from build123d import *

# Parameters (mm, degrees)
SKETCH4_R            = 55.88
BOSS_EXTRUDE2_DEPTH  = 10.16
BOSS_EXTRUDE4_DEPTH  = 101.6
BOSS_EXTRUDE5_DEPTH  = 9.525
BOSS_EXTRUDE6_START  = -9.525
BOSS_EXTRUDE6_DEPTH  = 9.525
CUT_EXTRUDE4_REACH   = 223.16
SKETCH12_R           = 21.5
SKETCH13_W           = 38.1
SKETCH13_H           = 69.85
CUT_EXTRUDE5_DEPTH   = 76.2
BOSS_EXTRUDE10_DEPTH = 19.05
SKETCH28_R           = 11.2395
CUT_EXTRUDE9_DEPTH   = 38.1
CUT_EXTRUDE10_DEPTH  = 7.366
CHAMFER1_SIZE        = 6.35
SKETCH30_R           = 2.1
CUT_EXTRUDE11_DEPTH  = 7.366
SKETCH31_R           = 3.175
CUT_EXTRUDE12_DEPTH  = 223.900333216
BOSS_EXTRUDE11_DEPTH = 38.1
CHAMFER2_SIZE        = 25.4
CUT_EXTRUDE13_REACH  = 233.204
SKETCH34_R           = 3.175
SKETCH35_R           = 3.175
CUT_EXTRUDE14_DEPTH  = 246.746626534
SKETCH36_W           = 63.5
SKETCH36_H           = 36.709955102
CUT_EXTRUDE15_DEPTH  = 63.5
FILLET1_R            = 6.35
SKETCH37_W           = 210.742334846
SKETCH37_H           = 201.224939079
CUT_EXTRUDE16_DEPTH  = 232.093968202


with BuildPart() as part:
    # Sketch4 → Boss-Extrude2 (new body)
    with BuildSketch(Plane(origin=(0, 0, 0), x_dir=(1, 0, 0), z_dir=(0, 1, 0))):
        with Locations(Location((0, 0, 0), (0, 0, 270))):
            Circle(SKETCH4_R)
    extrude(amount=BOSS_EXTRUDE2_DEPTH)

    # Sketch8 → Boss-Extrude4 (add)
    with BuildSketch(Plane(origin=(0, 10.16, 0), x_dir=(1, 0, 0), z_dir=(0, 1, 0))):
        Polygon((0, 43.994090512), (-38.1, 21.997045256), (-38.1, -21.997045256), (0, -43.994090512), (38.1, -21.997045256), (38.1, 21.997045256), align=None)
    extrude(amount=BOSS_EXTRUDE4_DEPTH)

    # Sketch9 → Boss-Extrude5 (add)
    with BuildSketch(Plane(origin=(-19.05, 0, -32.995567884), x_dir=(-0.8660254037844386, 0, 0.5000000000000003), z_dir=(-0.5000000000000002, 0, -0.8660254037844385))):
        with BuildLine():
            Line((21.997045256, 111.76), (-21.997045256, 111.76))
            Line((-21.997045256, 111.76), (-21.997045256, 124.225996336))
            ThreePointArc((-21.997045256, 124.225996336), (0, 188.144153123), (21.997045256, 124.225996336))
            Line((21.997045256, 124.225996336), (21.997045256, 111.76))
        make_face()
    extrude(amount=-BOSS_EXTRUDE5_DEPTH)

    # Sketch10 → Boss-Extrude6 (add)
    with BuildSketch(Plane(origin=(19.05, 0, 32.995567884), x_dir=(0.8660254037844386, 0, -0.5000000000000001), z_dir=(0.5000000000000001, 0, 0.8660254037844386)).offset(BOSS_EXTRUDE6_START)):
        with BuildLine():
            Line((-21.997045256, 111.76), (21.997045256, 111.76))
            Line((21.997045256, 111.76), (21.997045256, 124.225996336))
            ThreePointArc((21.997045256, 124.225996336), (0, 188.144153123), (-21.997045256, 124.225996336))
            Line((-21.997045256, 124.225996336), (-21.997045256, 111.76))
        make_face()
    extrude(amount=BOSS_EXTRUDE6_DEPTH)

    # Cut-Extrude4: up to this face of the body (flat: up to its plane)
    cut_extrude4_end = Plane(part.part.faces().sort_by_distance((19.05, 104.643172711, 32.995567884))[0])
    # Sketch12 → Cut-Extrude4 (cut, up to the picked face)
    with BuildSketch(Plane(origin=(-19.05, 0, -32.995567884), x_dir=(-0.8660254037844386, 0, 0.5000000000000003), z_dir=(-0.5000000000000002, 0, -0.8660254037844385)), mode=Mode.PRIVATE) as cut_extrude4_sk1:
        with Locations((0, 152.4)):
            Circle(SKETCH12_R)
    cut_extrude4_tool1 = split(extrude(cut_extrude4_sk1.sketch, amount=-CUT_EXTRUDE4_REACH, mode=Mode.PRIVATE), bisect_by=cut_extrude4_end, keep=Keep.BOTH, mode=Mode.PRIVATE)
    add(cut_extrude4_tool1.solids().sort_by(Axis((-19.05, 152.4, -32.995568), (0.5000000000000002, 0, 0.8660254037844385)))[0], mode=Mode.SUBTRACT)

    # Sketch13 → Cut-Extrude5 (cut, symmetric)
    with BuildSketch(Plane(origin=(-19.05, 0, 10.998522628), x_dir=(0.5000000000000002, 0, 0.8660254037844386), z_dir=(-0.8660254037844385, 0, 0.5000000000000001))):
        with Locations((0, 76.835)):
            Rectangle(SKETCH13_W, SKETCH13_H)
    extrude(amount=CUT_EXTRUDE5_DEPTH, both=True, mode=Mode.SUBTRACT)

    # Sketch22 → Boss-Extrude10 (add, symmetric)
    with BuildSketch(Plane(origin=(0, 0, 0), x_dir=(-0.8660254037844386, 0, 0.5000000000000001), z_dir=(-0.5000000000000001, 0, -0.8660254037844386))):
        with BuildLine():
            Line((43.994090512, 41.91), (102.10102108, 41.91))
            ThreePointArc((102.10102108, 41.91), (117.97602108, 26.035), (102.10102108, 10.16))
            Line((102.10102108, 10.16), (43.994090512, 10.16))
            Line((43.994090512, 10.16), (21.997045256, 10.16))
            Line((21.997045256, 10.16), (21.997045256, 41.91))
            Line((21.997045256, 41.91), (43.994090512, 41.91))
        make_face()
    extrude(amount=BOSS_EXTRUDE10_DEPTH, both=True)

    # Sketch28 → Cut-Extrude9 (cut)
    with BuildSketch(Plane(origin=(9.525, 0, 16.497783942), x_dir=(0.8660254037844386, 0, -0.5000000000000001), z_dir=(0.5000000000000001, 0, 0.8660254037844386))):
        with Locations((-102.10102108, 26.035)):
            Circle(SKETCH28_R)
    extrude(amount=-CUT_EXTRUDE9_DEPTH, mode=Mode.SUBTRACT)

    # Sketch29 → Cut-Extrude10 (cut)
    with BuildSketch(Plane(origin=(9.525, 0, 16.497783942), x_dir=(0.8660254037844386, 0, -0.5000000000000001), z_dir=(0.5000000000000001, 0, 0.8660254037844386))):
        with BuildLine():
            Line((-115.737415068, 17.907), (-109.863879848, 17.907))
            ThreePointArc((-109.863879848, 17.907), (-113.34052108, 26.035), (-109.863879848, 34.163))
            Line((-109.863879848, 34.163), (-115.737415068, 34.163))
            ThreePointArc((-115.737415068, 34.163), (-117.97602108, 26.035), (-115.737415068, 17.907))
        make_face()
    extrude(amount=-CUT_EXTRUDE10_DEPTH, mode=Mode.SUBTRACT)

    # Chamfer1
    chamfer1_edges = [part.edges().sort_by_distance(p)[0] for p in [
        (38.1, 41.91, -10.998522628),
        (28.575, 41.91, -27.49630657),
    ]]
    chamfer(chamfer1_edges, length=CHAMFER1_SIZE)

    # Sketch30 → Cut-Extrude11 (cut)
    with BuildSketch(Plane(origin=(0, 41.91, 0), x_dir=(1, 0, 0), z_dir=(0, 1, 0))):
        with Locations(Location((-88.422078008, -51.05051054, 0), (0, 0, 270))):
            Circle(SKETCH30_R)
    extrude(amount=-CUT_EXTRUDE11_DEPTH, mode=Mode.SUBTRACT)

    # Sketch31 → Cut-Extrude12 (cut, through all)
    with BuildSketch(Plane(origin=(0, 10.16, 0), x_dir=(1, 0, 0), z_dir=(0, 1, 0))):
        with Locations(Location((-49.089000823, 6.594762938, 0), (0, 0, 270))):
            Circle(SKETCH31_R)
        with Locations(Location((26.925278647, 41.57222955, 0), (0, 0, 270))):
            Circle(SKETCH31_R)
    cut_extrude12 = extrude(amount=-CUT_EXTRUDE12_DEPTH, mode=Mode.SUBTRACT)

    # Mirror1: Cut-Extrude12 across plane
    add(cut_extrude12.mirror(Plane(origin=(0, 0, 0), x_dir=(-0.8660254037844386, 0, 0.5000000000000001), z_dir=(-0.5000000000000001, 0, -0.8660254037844386))), mode=Mode.SUBTRACT)

    # Sketch33 → Boss-Extrude11 (add)
    with BuildSketch(Plane(origin=(0, 41.91, 0), x_dir=(1, 0, 0), z_dir=(0, 1, 0))):
        with BuildLine():
            Line((-43.411916389, -22.079834386), (-63.092428819, -33.442383535))
            Line((-63.092428819, -33.442383535), (-61.800298466, -35.680418955))
            Line((-61.800298466, -35.680418955), (-60.542722832, -37.858603849))
            Line((-60.542722832, -37.858603849), (-40.91541904, -26.504074545))
            ThreePointArc((-40.91541904, -26.504074545), (-33.742060338, -19.539834386), (-43.411916389, -22.079834386))
        make_face()
    extrude(amount=BOSS_EXTRUDE11_DEPTH)

    # Chamfer2
    chamfer2_edges = [part.edges().sort_by_distance(p)[0] for p in [
        (-61.817575825, 80.01, 35.650493692),
    ]]
    chamfer(chamfer2_edges, length=CHAMFER2_SIZE)

    # Cut-Extrude13: up to this plane
    cut_extrude13_end = Plane(origin=(-60.542722832, 80.01, 37.858603849), z_dir=(-0.500750644235671, 0, -0.8655915851587056))
    # Sketch34 → Cut-Extrude13 (cut, up to the surface)
    with BuildSketch(Plane(origin=(-1.292130352, 0, -2.23803542), x_dir=(-0.8660254037844386, 0, 0.5000000000000003), z_dir=(-0.5000000000000002, 0, -0.8660254037844385)), mode=Mode.PRIVATE) as cut_extrude13_sk1:
        with Locations((55.184849848, 61.159110234)):
            Circle(SKETCH34_R)
    cut_extrude13_tool1 = split(extrude(cut_extrude13_sk1.sketch, amount=-CUT_EXTRUDE13_REACH, mode=Mode.PRIVATE), bisect_by=cut_extrude13_end, keep=Keep.BOTH, mode=Mode.PRIVATE)
    add(cut_extrude13_tool1.solids().sort_by_distance((-49.083612, 61.15911, 25.35439))[0], mode=Mode.SUBTRACT)

    # Sketch35 → Cut-Extrude14 (cut, through all)
    with BuildSketch(Plane(origin=(19.05, 0, 32.995567884), x_dir=(0.8660254037844386, 0, -0.5000000000000001), z_dir=(0.5000000000000001, 0, 0.8660254037844386))):
        with Locations((0, 23.280078313)):
            Circle(SKETCH35_R)
    extrude(amount=-CUT_EXTRUDE14_DEPTH, mode=Mode.SUBTRACT)

    # Sketch36 → Cut-Extrude15 (cut, symmetric)
    with BuildSketch(Plane(origin=(-19.05, 0, 10.998522628), x_dir=(0.5000000000000004, 0, 0.8660254037844384), z_dir=(-0.8660254037844384, 0, 0.5000000000000004))):
        with Locations((0, 174.660846527)):
            Rectangle(SKETCH36_W, SKETCH36_H)
    extrude(amount=CUT_EXTRUDE15_DEPTH, both=True, mode=Mode.SUBTRACT)

    # Fillet1
    # the kernel refuses this fillet: 6.35 mm, written as the material it takes off along each edge
    with BuildSketch(Plane(origin=(12.272597523, 156.305868976, -21.027711652), x_dir=(0.04103819462533737, -0.9988766133891899, -0.023693412713994805), z_dir=(-0.5000000000000003, 0, -0.8660254037844386))) as fillet1_piece_1:
        with BuildLine():
            CenterArc((6.655634068, -6.291985478), FILLET1_R, 97.750867839, 84.965214409)
            Line((0.312767573, -6.592891819), (0, 0))
            ThreePointArc((0, 0), (2.899617679, -0.196427123), (5.799235358, 0))
        make_face()
    extrude(amount=19.675766287, mode=Mode.SUBTRACT)
    with BuildSketch(Plane(origin=(-24.346831236, 156.305868976, 0.114525399), x_dir=(-0.04103819462533767, -0.9988766133891899, 0.023693412713994975), z_dir=(-0.5000000000000003, 0, -0.8660254037844386))) as fillet1_piece_2:
        with BuildLine():
            CenterArc((6.655634068, 6.291985478), FILLET1_R, 177.283917752, 84.965214409)
            Line((0.312767573, 6.592891819), (0, 0))
            ThreePointArc((0, 0), (2.899617679, 0.196427123), (5.799235358, 0))
        make_face()
    extrude(amount=19.675766287, mode=Mode.SUBTRACT)
    with BuildSketch(Plane(origin=(-14.894977291, 156.305868976, 45.261361242), x_dir=(-0.011364190914464473, -0.999913899736612, 0.0065611186835884), z_dir=(-0.5000000000000002, 0, -0.8660254037844386)), Plane(origin=(-36.459231913, 156.305868976, 7.91097661), x_dir=(-0.011364190914463116, -0.999913899736612, 0.0065611186835876165), z_dir=(-0.5000000000000002, 0, -0.8660254037844386))) as fillet1_piece_3:
        with BuildLine():
            CenterArc((6.26760006, -6.320536654), FILLET1_R, 84.478464497, 94.769665105)
            Line((-0.081853204, -6.237210446), (0, 0))
            ThreePointArc((0, 0), (3.439298151, 0.165849191), (6.878596303, 0))
        make_face()
    extrude(amount=20.371490756, mode=Mode.SUBTRACT)
    with BuildSketch(Plane(origin=(25.080722669, 156.305868976, -27.619132734), x_dir=(0.011364190914465366, -0.999913899736612, -0.00656111868358885), z_dir=(-0.5000000000000002, 0, -0.8660254037844386)), Plane(origin=(46.644977291, 156.305868976, 9.731251898), x_dir=(0.011364190914466365, -0.999913899736612, -0.006561118683589426), z_dir=(-0.5000000000000002, 0, -0.8660254037844386))) as fillet1_piece_4:
        with BuildLine():
            CenterArc((6.26760006, 6.320536654), FILLET1_R, 180.751870398, 94.769665105)
            Line((-0.081853204, 6.237210446), (0, 0))
            ThreePointArc((0, 0), (3.439298151, -0.165849191), (6.878596303, 0))
        make_face()
    extrude(amount=20.371490756, mode=Mode.SUBTRACT)

    # Sketch37 → Cut-Extrude16 (cut, through all)
    with BuildSketch(Plane(origin=(0, 0, 0), x_dir=(-0.8660254037844386, 0, 0.5000000000000001), z_dir=(-0.5000000000000001, 0, -0.8660254037844386))):
        with Locations((30.487295463, 97.29801522)):
            Rectangle(SKETCH37_W, SKETCH37_H)
    extrude(amount=-CUT_EXTRUDE16_DEPTH, mode=Mode.SUBTRACT)


solid = part.part
Work out the finished part from the listing and answer in its coordinate system (mm). A direction names the side the tool comes from. Give positions to 0.01 mm unless a question says otherwise; leave off trailing zeros. Order: outer loops, then holes, each group sorted by start corner. A loop starts at its lowest first (then second) coordinate and runs counter-clockwise, first axis right, second up. Notation, with made-up numbers: (85.5, 44.25) - (138.5, 44.25) arc R20 cw to (138.5, 71.25) - close; hole circle Ø4 at (31, -36). An arc over 180 degrees is marked (long way). Answer as CSV lines item,"result". Start each with the question number.
Q1. For faces 1 (the face through (-14.72, 129.395, -24.497)), 2 (the face through (-38, 80.01, 19)), 3 (the face through (-50.93, 55.44, 26.42)), 4 (the face through (-39.489, 60.693, 17.064)), determine the directions among +Z, -Z, +X, -X, +Y, -Y from which every point of the face is accessible in a straight line to the end or side of a thin tool.
Q2. The part is cut by section C-C (x = 34). Write down the section's boundary in (y, z).
Q3. The part is cut by section B-B (y = 115.5). Write down the section's boundary in (x, z).
Q4. The mould has two halves that part along X. Classify faces 5 (the face through (-26.869, 5.009, -48.996)), 6 (the face through (-106.996, 26.384, 50.622)), 7 (the face through (-45.94, 5.15, -7.01)): +X half, -X half, draft (parallel to the pull), parting line (faces both ways), or undercut.
Q5. The part is cut by section D-D (y = 167). Write down the section's boundary in (x, z).
Q6. Find the intervals of material crossed by L1, parallel to Y at x = -42.5, z = -16.5; L2, parallel to Y at x = -54, z = -9.5; L3, parallel to Y at x = -14.5, z = -9.5, in increasing order. Write a range as [from, to].
Q7. Given pin 1 Ø2.5 at (x, z) = (-40, -11.5) entering from +Y; pin 2 Ø3 at (y, z) = (46, 22) entering from -X; pin 3 Ø5 at (y, z) = (32.5, 42) entering from -X, each flat-ended and moving along its own axis, determine where each tip first touches the part or whether it passes through.
Q8. The part is cut by section A-A (y = 73). Write down the section's boundary in (x, z).
Check result:
1,face 1,"+Z, +X, +Y"
1,face 2,"+Z, +X, -X, +Y"
1,face 3,"-Z, -X, +Y"
1,face 4,"+Y"
2,outline,"(0, -44.35) - (10.16, -44.35) - (10.16, -24.36) - (35.56, -24.36) - (39.66, -19.63) - (0, -19.63) - close"
3,outline,"(-38.1, -22) - (0, -43.99) - (4.76, -35.75) - (-33.34, -13.75) - close"
4,face 5,"parting line"
4,face 6,"-X half"
4,face 7,"undercut"
5,outline,"(-47.31, -16.68) - (-32.72, -25.1) - (-29.54, -19.61) - (-44.13, -11.18) - close; (-5.38, -40.89) - (9.21, -49.31) - (12.38, -43.81) - (-2.21, -35.39) - close"
6,L1,"y = [0, 10.16], [130.9, 173.9]"
6,L2,"y = [0, 10.16]"
6,L3,"y = [0, 41.91]"
7,pin 1,"stops at y = 156.31"
7,pin 2,"stops at x = -45.87"
7,pin 3,"stops at x = -111.26"
8,outline,"(-47.17, 24.25) - (-43.41, 22.08) arc R5.17 ccw to (-33.77, 19.5) - (-45.87, 26.49) - close; (-38.1, -22) - (0, -43.99) - (19.05, -33) - (-38.1, 0) - close"
